```python
from build123d import *

# Parameters (mm, degrees)
F1_DEPTH    = 63.5
F2_DEPTH    = 25.4
F3_DEPTH    = 7.9375
F5_T1_DEPTH = 57.15


# Not quite as in the source:
# - a fillet or chamfer that OpenCascade refuses, or shapes differently, is made with other operations: its cross-section is extruded or revolved along the edge and cut away or added


with BuildPart() as f1:
    # F0 (on Front) → F1 (new body, symmetric)
    with BuildSketch(Plane.XZ):
        Polygon((-41.275, 9.525), (-41.275, -9.525), (41.275, -9.525), (41.275, 9.525), (22.225, 9.525), align=None)
    extrude(amount=F1_DEPTH, both=True)

    # F0 (on Front) → F2 (join, symmetric)
    with BuildSketch(Plane.XZ):
        with BuildLine():
            Line((22.225, 9.525), (41.275, 9.525))
            Line((41.275, 9.525), (41.275, 27.0002))
            ThreePointArc((41.275, 27.0002), (45.4000764986, 37.6751671059), (55.631525696, 42.8024106298))
            Line((55.631525696, 42.8024106298), (55.631525696, 61.8921741601))
            ThreePointArc((55.631525696, 61.8921741601), (31.9231458554, 51.1530767431), (22.225, 27.0002))
            Line((22.225, 27.0002), (22.225, 9.525))
        make_face()
        with BuildLine():
            ThreePointArc((57.15, 61.9252), (56.3905832965, 61.9169425639), (55.631525696, 61.8921741601))
            Line((55.631525696, 61.8921741601), (55.631525696, 42.8024106298))
            ThreePointArc((55.631525696, 42.8024106298), (56.3898910433, 42.8569922158), (57.15, 42.8752))
            Line((57.15, 42.8752), (84.0459217609, 42.8752))
            Line((84.0459217609, 42.8752), (84.1045851677, 61.9252))
            Line((84.1045851677, 61.9252), (57.15, 61.9252))
        make_face()
    extrude(amount=F2_DEPTH, both=True)

    # F0 (on Front) → F3 (join, symmetric)
    with BuildSketch(Plane.XZ):
        with BuildLine():
            add(Edge.make_bspline(
                [(-41.275, 9.525), (-0.4847672351, 18.3894253248), (13.3813129593, 64.201731175), (55.631525696, 62.0233434816)],
                knots=[0, 0, 0, 0, 110.1949360256, 110.1949360256, 110.1949360256, 110.1949360256], degree=3))
            Line((-41.275, 9.525), (22.225, 9.525))
            Line((22.225, 9.525), (22.225, 27.0002))
            ThreePointArc((22.225, 27.0002), (31.9231458554, 51.1530767431), (55.631525696, 61.8921741601))
            Line((55.631525696, 61.8921741601), (55.631525696, 62.0233434816))
        make_face()
    extrude(amount=F3_DEPTH, both=True)

    # F0 (on Front) → F4 (revolve)
    with BuildSketch(Plane.XZ):
        Polygon((106.431525696, 66.675), (84.1192119104, 66.675), (84.1045851677, 61.9252), (84.0459217609, 42.8752), (84.0312168002, 38.1), (106.431525696, 38.1), align=None)
    revolve(axis=Axis((84.0752143553, 0, 52.3875), (0.0030794293, 0, 0.9999952585)))

    # F5: fillet of radius 7.62 on 4 edges, made by hand

    # F5_s2 → F5_t1 (cut)
    with BuildSketch(Plane.XY.offset(-28.575)):
        with BuildLine():
            add(Edge.make_bspline(
                [(-41.275, -55.88), (-41.275, -63.5), (-33.655, -63.5)],
                knots=[0, 0, 0, 1, 1, 1], degree=2, weights=[1, 1, 1]))
            Line((-33.655, -63.5), (-41.275, -63.5))
            Line((-41.275, -63.5), (-41.275, -55.88))
        make_face()
        with BuildLine():
            add(Edge.make_bspline(
                [(33.655, -63.5), (41.275, -63.5), (41.275, -55.88)],
                knots=[0, 0, 0, 1, 1, 1], degree=2, weights=[1, 1, 1]))
            Line((41.275, -55.88), (41.275, -63.5))
            Line((41.275, -63.5), (33.655, -63.5))
        make_face()
        with BuildLine():
            add(Edge.make_bspline(
                [(-41.275, 55.88), (-41.275, 63.5), (-33.655, 63.5)],
                knots=[0, 0, 0, 1, 1, 1], degree=2, weights=[1, 1, 1]))
            Line((-33.655, 63.5), (-41.275, 63.5))
            Line((-41.275, 63.5), (-41.275, 55.88))
        make_face()
        with BuildLine():
            add(Edge.make_bspline(
                [(33.655, 63.5), (41.275, 63.5), (41.275, 55.88)],
                knots=[0, 0, 0, 1, 1, 1], degree=2, weights=[1, 1, 1]))
            Line((41.275, 55.88), (41.275, 63.5))
            Line((41.275, 63.5), (33.655, 63.5))
        make_face()
    extrude(amount=F5_T1_DEPTH, mode=Mode.SUBTRACT)


solid = f1.part
```
Design review of the part built by this model. Coordinates are the model's own, in mm. A direction names the side the tool comes from. Give positions to 0.01 mm unless a question says otherwise; leave off trailing zeros. Order: outer loops, then holes, each group sorted by start corner. A loop starts at its lowest first (then second) coordinate and runs counter-clockwise, first axis right, second up. Notation, with made-up numbers: (3, 54) -> (18, 54) arc R30 cw to (18, 77) -> close; hole circle Ø7 at (-7.75, 89.25). An arc over 180 degrees is marked (long way). Write item = value, one per line. Start each with the question number.
(1) To check wall thickness, follow line 1 along X through (y, z) = (-21, 23.5) (3 decimals); line 2 along Z through (x, y) = (-6.5, -30.5) (3 decimals); line 3 along Z through (x, y) = (63, 5). State the ranges of each line that lie inside material, in increasing order.
(2) For pin 1 (15.5 mm diameter, centred on x = 61.5, z = 33, fed in from +Y); pin 2 (1 mm diameter, centred on y = 9, z = 7, fed in from +X) (3 decimals); pin 3 (14 mm diameter, centred on y = 16.5, z = 17.5, fed in from -X) (3 decimals), all flat-tipped, find the tip position at first contact; note any pin that passes through.
(3) For faces 4 (the face through (22.225, 17, 18)), 5 (the face through (22.225, -17, 18)), 6 (the face through (46, -25.4, 42)), list the 3-axis set-ups (+Z, -Z, +X, -X, +Y, -Y) from which the entire face can be reached by the end or side of a thin tool; tool diameter is ignored.
(4) We need section A-A on y = -45. Write out the cut boundary in (x, z) (3 decimals).
(5) Mouldability with a two-part tool opening along X and no side actions: class faces 1 (the face through (0, -63.5, 0)), 2 (the face through (-41.275, -1, 0)), 3 (the face through (45.8, -0.4, 38.1)) as +X half, -X half, draft (parallel to the pull), parting line (faces both ways), or undercut.
Numbers:
q1.line_1 = 22.225 to 41.275
q1.line_2 = -9.525 to 9.525
q1.line_3 = 38.23 to 66.81
q2.pin_1 = 14.81
q2.pin_2 = 41.275
q2.pin_3 = 22.225
q3.face_4 = +Z, -X, +Y
q3.face_5 = +Z, -X, -Y
q3.face_6 = +Z, +X, -X, -Y
q4.outline = (-41.275, -9.525) -> (41.275, -9.525) -> (41.275, 9.525) -> (-41.275, 9.525) -> close
q5.face_1 = draft
q5.face_2 = -X half
q5.face_3 = undercut
